Part print with two shaded views. Sizes in mm from the minimum x, y, z corner. Round coordinates to 2 decimals unless told otherwise and drop trailing zeros. Write each loop counter-clockwise with the first axis right and the second up, starting at its lowest first coordinate (ties: lowest second). Pieces come first, ordered by that corner, then holes. Notation, with made-up numbers: (-18.75, -18.5) -> (-9.75, -18.5) arc R19 cw to (-9.75, 8.5) -> close; hole circle Ø7 at (73.5, -15). An arc over 180 degrees is marked (long way). Return JSON: item names as keys, results as strings.
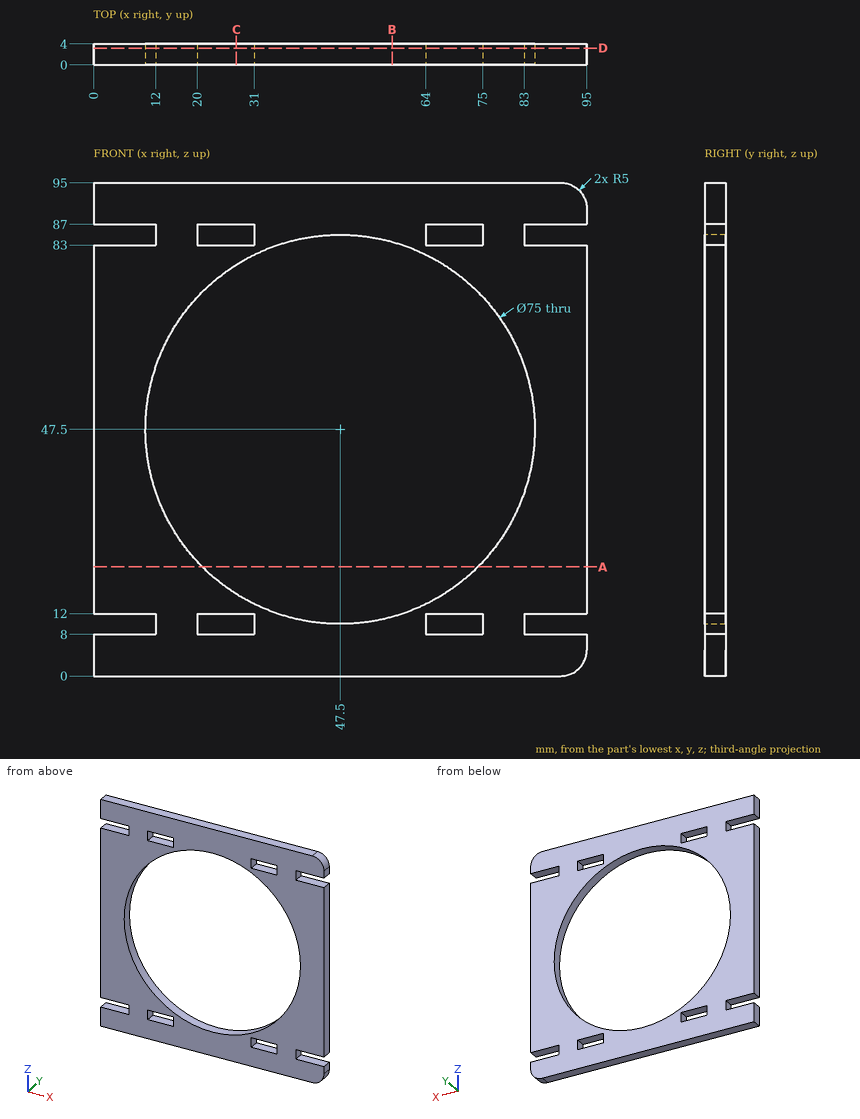
Q1. Saw through at B-B on x = 57.5. List the corners of the cut face in (y, z).
Verdict:
{"outline": "(0, 0) -> (4, 0) -> (4, 11.36) -> (0, 11.36) -> close; (0, 83.64) -> (4, 83.64) -> (4, 95) -> (0, 95) -> close"}
Q2. Saw through at A-A on z = 21. List the corners of the cut face in (x, y).
Verdict:
{"outline": "(0, 0) -> (20.97, 0) -> (20.97, 4) -> (0, 4) -> close; (74.03, 0) -> (95, 0) -> (95, 4) -> (74.03, 4) -> close"}
Q3. Saw through at C-C on x = 27.5. List the corners of the cut face in (y, z).
Verdict:
{"outline": "(0, 0) -> (4, 0) -> (4, 8) -> (0, 8) -> close; (0, 12) -> (4, 12) -> (4, 15.78) -> (0, 15.78) -> close; (0, 79.22) -> (4, 79.22) -> (4, 83) -> (0, 83) -> close; (0, 87) -> (4, 87) -> (4, 95) -> (0, 95) -> close"}
Q4. Saw through at D-D on y = 3.2. Count the separate pieces of the cut face and the enclosed holes in it, then the cut area to 3 significant figures.
Verdict:
{"separate pieces": "1", "enclosed holes": "5", "area": "4,230 mm²"}
Q5. Wall check: L1, parallel to Z at x = 5, y = 2; L2, parallel to X at y = 2.2, z = 47.5; L3, parallel to X at y = 3.3, z = 9. Give the ranges that are in metal, low to high.
Verdict:
{"L1": "z = 0 to 8, 12 to 83, 87 to 95", "L2": "x = 0 to 10, 85 to 95", "L3": "x = 12 to 20, 31 to 64, 75 to 83"}
Q6. Pin check, flat tip, straight feed: pin 1 Ø1.2 at (x, y) = (91, 1) entering from -Z. Stop position of the tip, or through.
Verdict:
{"pin 1": "stops at z = 0.02"}
